from build123d import *

# Parameters (mm, degrees)
BOSS_EXTRUDE1_DEPTH            = 3.175
CUT_EXTRUDE1_REACH             = 5.252
SKETCH2_R                      = 1.6256
CUT_EXTRUDE1_DIRECTION_2_DEPTH = 4.175


with BuildPart() as part:
    # Sketch1 → Boss-Extrude1 (new body, symmetric)
    with BuildSketch(Plane(origin=(0, 0, 0), x_dir=(0, 0, -1), z_dir=(1, 0, 0))):
        with BuildLine():
            Line((-10.16, 0), (-4.259709497, 0))
            ThreePointArc((-4.259709497, 0), (-3.50073933, 0.251734668), (-3.042649641, 0.907142857))
            ThreePointArc((-3.042649641, 0.907142857), (0, 3.175), (3.042649641, 0.907142857))
            ThreePointArc((3.042649641, 0.907142857), (3.50073933, 0.251734668), (4.259709497, 0))
            Line((4.259709497, 0), (10.16, 0))
            ThreePointArc((10.16, 0), (10.488700187, -0.043274201), (10.795, -0.170147737))
            Line((10.795, -0.170147737), (12.994704526, -1.440147737))
            Line((12.994704526, -1.440147737), (13.544630657, -1.757647737))
            ThreePointArc((13.544630657, -1.757647737), (13.608067425, -1.275797644), (13.312204526, -0.890221606))
            Line((13.312204526, -0.890221606), (11.1125, 0.379778394))
            ThreePointArc((11.1125, 0.379778394), (10.653050281, 0.570088699), (10.16, 0.635))
            Line((10.16, 0.635), (4.709286039, 0.635))
            ThreePointArc((4.709286039, 0.635), (3.999334456, 0.851971629), (3.531964529, 1.42875))
            ThreePointArc((3.531964529, 1.42875), (0, 3.81), (-3.531964529, 1.42875))
            ThreePointArc((-3.531964529, 1.42875), (-3.999334456, 0.851971629), (-4.709286039, 0.635))
            Line((-4.709286039, 0.635), (-10.16, 0.635))
            ThreePointArc((-10.16, 0.635), (-10.889011939, 0.489990509), (-11.507038418, 0.077038418))
            Line((-11.507038418, 0.077038418), (-13.292936294, -1.708859457))
            ThreePointArc((-13.292936294, -1.708859457), (-13.48919858, -2.160845652), (-13.303204425, -2.6171532))
            Line((-13.303204425, -2.6171532), (-12.854076836, -2.168025612))
            Line((-12.854076836, -2.168025612), (-11.058025612, -0.371974388))
            ThreePointArc((-11.058025612, -0.371974388), (-10.646007959, -0.096672994), (-10.16, 0))
        make_face()
    extrude(amount=BOSS_EXTRUDE1_DEPTH, both=True)

    # Sketch2 → Cut-Extrude1 (cut, up to next)
    with BuildSketch(Plane(origin=(0, 0.635, 0), x_dir=(1, 0, 0), z_dir=(0, 1, 0)), mode=Mode.PRIVATE) as cut_extrude1_sk1:
        with Locations((0, -7.73176)):
            Circle(SKETCH2_R)
    cut_extrude1_tool1 = extrude(cut_extrude1_sk1.sketch, amount=-CUT_EXTRUDE1_REACH, mode=Mode.PRIVATE) & part.part
    add(cut_extrude1_tool1.solids().sort_by_distance((0, 0.635, 7.73176))[0], mode=Mode.SUBTRACT)
    # Sketch2 → Cut-Extrude1 (cut, up to next)
    with BuildSketch(Plane(origin=(0, 0.635, 0), x_dir=(1, 0, 0), z_dir=(0, 1, 0)), mode=Mode.PRIVATE) as cut_extrude1_sk2:
        with Locations((0, 7.91718)):
            Circle(SKETCH2_R)
    cut_extrude1_tool2 = extrude(cut_extrude1_sk2.sketch, amount=-CUT_EXTRUDE1_REACH, mode=Mode.PRIVATE) & part.part
    add(cut_extrude1_tool2.solids().sort_by_distance((0, 0.635, -7.91718))[0], mode=Mode.SUBTRACT)

    # Sketch2 → Cut-Extrude1 direction 2 (cut)
    with BuildSketch(Plane(origin=(0, 0.635, 0), x_dir=(1, 0, 0), z_dir=(0, 1, 0))):
        with Locations((0, -7.73176)):
            Circle(SKETCH2_R)
        with Locations((0, 7.91718)):
            Circle(SKETCH2_R)
    extrude(amount=CUT_EXTRUDE1_DIRECTION_2_DEPTH, mode=Mode.SUBTRACT)


solid = part.part
Could you check a few things on this model? Use its own coordinates, in mm. A direction names the side the tool comes from. Give positions to 0.01 mm unless a question says otherwise; leave off trailing zeros. Order: outer loops, then holes, each group sorted by start corner. A loop starts at its lowest first (then second) coordinate and runs counter-clockwise, first axis right, second up. Notation, with made-up numbers: (-37.75, -10.75) -> (-6.75, -10.75) arc R31 ccw to (-6.75, 25.25) -> close; hole circle Ø8 at (27, 40). An arc over 180 degrees is marked (long way). Return JSON: item names as keys, results as strings.
1. On a 3-axis mill with a long thin cutter (end or side, diameter ignored), from which of +Z, -Z, +X, -X, +Y, -Y can I reach the whole of each face in a straight line? I mean faces 1 (the cylindrical face through (0.044, 0.245, 3.51)), 2 (the flat face through (0, 0.635, -6)), 3 (the flat face through (1, 0.635, 6)). Say none if no direction works.
Answer list:
{"face 1": "+X, -X, -Y", "face 2": "-Z, +X, -X, +Y", "face 3": "+Z, +X, -X, +Y"}
2. Imagine slicing it at B-B on z = 8.25. List the corners of the cut face in (x, y) for me (3 decimals), then the cut area to 3 significant figures.
Answer list:
{"outline": "(-3.175, 0) -> (-1.541, 0) -> (-1.541, 0.635) -> (-3.175, 0.635) -> close; (1.541, 0) -> (3.175, 0) -> (3.175, 0.635) -> (1.541, 0.635) -> close", "area": "2.08 mm2"}
3. Imagine slicing it at C-C on y = 2. List the corners of the cut face in (x, z) for me (3 decimals).
Answer list:
{"outline": "(-3.175, -3.243) -> (3.175, -3.243) -> (3.175, -2.466) -> (-3.175, -2.466) -> close; (-3.175, 2.466) -> (3.175, 2.466) -> (3.175, 3.243) -> (-3.175, 3.243) -> close"}
4. Thinking about a two-plate mould opening in Z: for faces 4 (the cylindrical face through (0.04, 0.26, -3.49)), 5 (the cylindrical face through (0.04, -1.28, -13.61)), 6 (the cylindrical face through (0.04, -2.15, 13.49)), which applies, pulls with the +Z half, pulls with the -Z half, needs draft (parallel to the pull), parting line crosses it, or undercut?
Answer list:
{"face 4": "undercut", "face 5": "pulls with the -Z half", "face 6": "pulls with the +Z half"}
5. For pin 1 Ø1.8 at (x, z) = (-0.5, -8.5) entering from -Y; pin 2 Ø2 at (y, z) = (-1.5, -2) entering from +X; pin 3 Ø1.5 at (x, y) = (1, 3) entering from +Z, each with a flat end and sliding along its axis, tell me the tip position at first contact or that it passes through.
Answer list:
{"pin 1": "stops at y = 0", "pin 2": "passes through", "pin 3": "stops at z = 3.07"}
6. I need wall thicknesses on line 1 (Z direction, x = 0, y = 0.4); line 2 (Z direction, x = 0, y = 0.15); line 3 (Z direction, x = -2.25, y = -1). Which ranges of each line are inside material? Lowest first, please. Write a range as from..to.
Answer list:
{"line 1": "z = -11.08..-9.54, -6.29..-3.33, 3.33..6.11, 9.36..11.08", "line 2": "z = -11.51..-9.54, -6.29..-3.66, 3.66..6.11, 9.36..11.43", "line 3": "z = -13.45..-12.23, 11.69..12.58"}
7. Imagine slicing it at A-A on x = 0. Give the number of separate pieces and of enclosed holes in the cut face, then the cut area to 3 significant figures.
Answer list:
{"separate pieces": "3", "enclosed holes": "0", "area": "16.0 mm2"}
